Geometry: see drawing. Coordinates: mm, zero at the bounding-box minimum. A direction names the side the tool comes from. Coordinates: 2 decimals unless noted, no trailing zeros. Loops run counter-clockwise (first coordinate to the right, second up) from the corner with the lowest first, then second, coordinate; pieces in that order, holes last. Notation, with made-up numbers: (34, 57) - (88, 57) arc R13 cw to (88, 77) - close; hole circle Ø9 at (-26.5, 50.25). An arc over 180 degrees is marked (long way). Use a Markdown table: item, result. Add a question column.
1. Section query A-A on z = 3. Return the cut outline in (x, y).
2. Section query B-B on x = 1.6. Return the cut outline in (y, z).
3. Ray query, L1, parallel to Y at x = 1.95, z = 1; L2, parallel to X at y = 0.1, z = 7; L3, parallel to Z at x = 1.05, y = 1.5. Return the intervals inside material, ascending. Write a range as [from, to].
4. Contact query for flat-ended pins moving along their axis: P1, Ø1, axis at x = 2, z = 1.5, coming from the -Y side; P2, Ø1.6, axis at x = 1, z = 3.5, coming from the -Y side. Output: stop coordinate, or through.
5. Access query for the marked faces 1 and 2. Directions: +Z, -Z, +X, -X, +Y, -Y. A direction counts if a zero-diameter tool reaches every point of the face in a straight line with its end or side. Return the directions, or none.
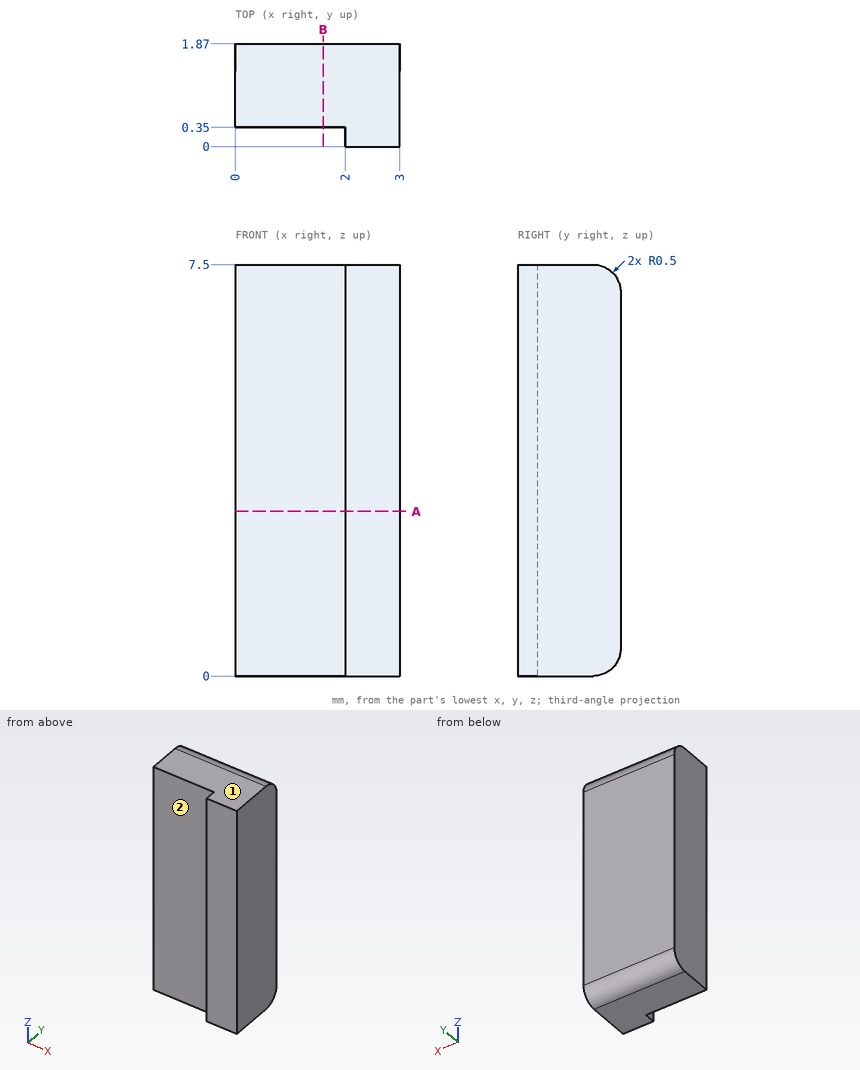
Resolved:
| question | item | result |
|---|---|---|
| 1 | outline | (0, 0.35) - (2, 0.35) - (2, 0) - (3, 0) - (3, 1.87) - (0, 1.87) - close |
| 2 | outline | (0.35, 0) - (1.37, 0) arc R0.5 ccw to (1.87, 0.5) - (1.87, 7) arc R0.5 ccw to (1.37, 7.5) - (0.35, 7.5) - close |
| 3 | L1 | [0.35, 1.87] |
| 3 | L2 | [2, 3] |
| 3 | L3 | [0.02, 7.48] |
| 4 | P1 | y = 0 |
| 4 | P2 | y = 0.35 |
| 5 | face 1 | +Z, +X, -X, +Y, -Y |
| 5 | face 2 | +Z, -Z, -X, -Y |
